```python
from build123d import *

# Parameters (mm, degrees)
SKETCH1_W                      = 330.2
SKETCH1_H                      = 203.2
BOSS_EXTRUDE1_DEPTH            = 6.35
F_1_4_0_25_PRESS_DOWEL_HOLE1_D = 6.35
M8X1_0_TAPPED_HOLE1_D          = 7


with BuildPart() as part:
    # Sketch1 → Boss-Extrude1 (new body)
    with BuildSketch(Plane(origin=(0, 0, 0), x_dir=(1, 0, 0), z_dir=(0, 1, 0))):
        Rectangle(SKETCH1_W, SKETCH1_H)
    extrude(amount=BOSS_EXTRUDE1_DEPTH)

    # 1/4 (0.25) Press Dowel Hole1 (through all)
    with Locations(Plane(origin=(0, 6.35, 0), x_dir=(1, 0, 0), z_dir=(0, 1, 0))):
        with Locations((-140.85176751, 38.099999999), (-140.851357678, -38.099999999), (-48.715925188, -38.099504462), (-48.715925188, 38.100495539), (45.083869896, 38.101000028), (45.084279728, -38.098999971)):
            Hole(F_1_4_0_25_PRESS_DOWEL_HOLE1_D / 2)

    # M8x1.0 Tapped Hole1 (through all)
    with Locations(Plane(origin=(0, 6.35, 0), x_dir=(1, 0, 0), z_dir=(0, 1, 0))):
        with Locations((-140.851562594, 82.55), (-48.715925188, 82.55), (45.084074812, 76.701000029), (45.084074812, -76.698999971), (-48.715925188, -82.55), (-140.851562594, -82.55), (139.954074812, 57.072042721), (139.954074812, -57.072042721)):
            Hole(M8X1_0_TAPPED_HOLE1_D / 2)


solid = part.part
```
Input: part model. Units: mm. Frame: model coordinates. Round coordinates to 2 decimals unless told otherwise and drop trailing zeros. Write each question's results on one line, items separated by ' | '.
1. Mould query, pull axis X, two halves, no side actions, for faces 1 (the face through (48.256, 3.131, -38.241)), 2 (the face through (165.1, 3, 1)), 3 (the face through (-2, 6.35, -1)). Classes: +X half, -X half, draft (parallel to the pull), parting line (faces both ways), or undercut.
Geometry results:
face 1: undercut | face 2: +X half | face 3: draft
2. First-contact query: P1, Ø10, axis at x = -140.85, z = -38.1, coming from the +Y side. Flat tip, straight axial feed; report the tip coordinate or a pass-through.
Geometry results:
P1: y = 6.35
3. Ray query, line 1 (X direction, y = 2.5, z = -77); line 2 (X direction, y = 3.75, z = -37.5); line 3 (X direction, y = 1.75, z = 82.55). Return the intervals inside material, ascending. Write a range as from..to.
Geometry results:
line 1: -165.1..41.6, 48.57..165.1 | line 2: -165.1..-143.97, -137.73..-51.83, -45.6..41.97, 48.2..165.1 | line 3: -165.1..-144.35, -137.35..-52.22, -45.22..165.1
